```python
from build123d import *

# Parameters (mm, degrees)
BOSS_EXTRU_1_DEPTH = 32
CHANFREIN1_SIZE    = 1.5


with BuildPart() as part:
    # Esquisse1 → Boss.-Extru.1 (new body)
    with BuildSketch(Plane.XY):
        Polygon((-4, 0), (4, 0), (4, -2), (2.5, -3.5), (-2.5, -3.5), (-4, -2), align=None)
    extrude(amount=BOSS_EXTRU_1_DEPTH)

    # Chanfrein1
    chanfrein1_edges = [part.edges().sort_by_distance(p)[0] for p in [
        (0, -3.5, 0),
        (0, -3.5, 32),
    ]]
    chamfer(chanfrein1_edges, length=CHANFREIN1_SIZE)


solid = part.part
```
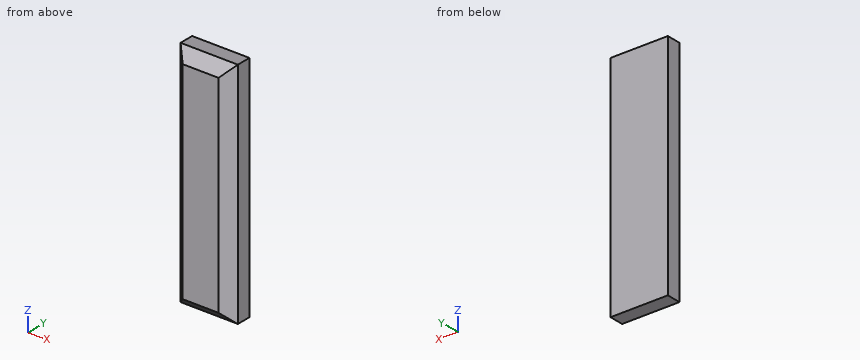
The listing builds one solid part. Answer for the finished solid, in the listing's coordinates (mm). Give positions to 0.01 mm unless a question says otherwise; leave off trailing zeros. Write each loop counter-clockwise with the first axis right and the second up, starting at its lowest first coordinate (ties: lowest second). Pieces come first, ordered by that corner, then holes. Notation, with made-up numbers: (58, 70.5) - (73, 70.5) arc R34 cw to (73, 102.5) - close; hole circle Ø2 at (10, 64.25). An arc over 180 degrees is marked (long way). Use one line per item in the form item = value. Start each with the question number.
1) Find section A-A on z = 22. Determine the outline of the cut face in (x, y), plus the area to 4 significant figures.
2) Find section C-C on y = -2.75. Determine the outline of the cut face in (x, z), plus the area to 3 significant figures.
3) Consider line 1 along Y through (x, z) = (3.5, 15); line 2 along X through (y, z) = (-2.6, 4); line 3 along Y through (x, z) = (3, 14.5). Determine where each line is inside the solid, lowest interval first. Write a range as from..to.
4) Find section B-B on x = -0.5. Determine the outline of the cut face in (y, z).
Geometry results:
q1.outline = (-4, -2) - (-2.5, -3.5) - (2.5, -3.5) - (4, -2) - (4, 0) - (-4, 0) - close
q1.area = 25.75 mm2
q2.outline = (-3.25, 0.75) - (3.25, 0.75) - (3.25, 31.25) - (-3.25, 31.25) - close
q2.area = 198 mm2
q3.line_1 = -2.5..0
q3.line_2 = -3.4..3.4
q3.line_3 = -3..0
q4.outline = (-3.5, 1.5) - (-2, 0) - (0, 0) - (0, 32) - (-2, 32) - (-3.5, 30.5) - close
